Build history of the part. All positions in model axes, mm. Face numbers are marked on the shaded views. A direction names the side the tool comes from. Give positions to 0.01 mm unless a question says otherwise; leave off trailing zeros. Order: outer loops, then holes, each group sorted by start corner. A loop starts at its lowest first (then second) coordinate and runs counter-clockwise, first axis right, second up. Notation, with made-up numbers: (44, 34.5) -> (65, 34.5) arc R14 cw to (65, 43.5) -> close; hole circle Ø7 at (6.5, 60). An arc over 180 degrees is marked (long way). One line per question, with ' | ' between items. Start each with the question number.
(1) Pull direction X, two halves, no side cores. Call the marked faces 1, 2 and 3: +X half, -X half, draft (parallel to the pull), parting line (faces both ways), or undercut.
(2) Cut at C-C (y = -140). Give the cut face in (x, z), then the cut area to 3 significant figures.
(3) Drill centre lines: L1, parallel to Z at x = 10, y = -161; L2, parallel to Z at x = -1, y = -193.5. Where is each one in solid material? Low to high. Write a range as from..to.
(4) Pin check, flat tip, straight feed: pin 1 Ø2 at (x, z) = (-4, 16) entering from +Y. Stop position of the tip, or through.
(5) Which spindle directions (+Z, -Z, +X, -X, +Y, -Y) get a long thin tool onto all of the face, cutting with end or side? Do the marked faces 4 and 5. Say none if no direction does.
(6) Cut at A-A (z = 2). Give the cut face in (x, y).
(7) Cut at B-B (x = -8). Give the cut face in (y, z), then the cut area to 3 significant figures.
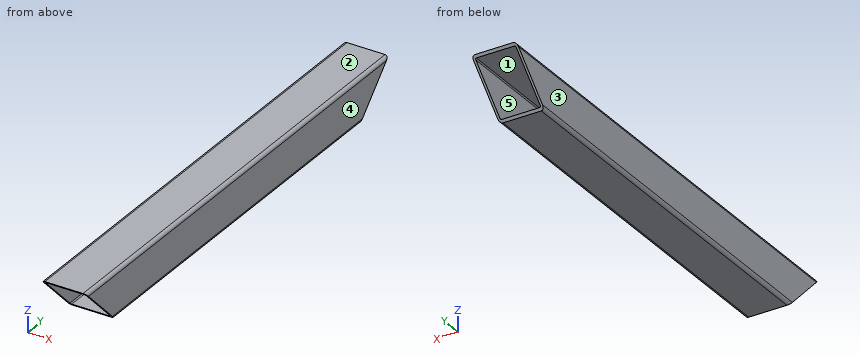
from build123d import *

# Parameters (mm, degrees)
F2_W     = 40
F2_H     = 40
F3_DEPTH = 214
F4_R     = 3
F5_T     = -2
F7_DEPTH = 40.001
F9_DEPTH = 40.001


with BuildPart() as f3:
    # F2 (on Front) → F3 (new body, symmetric)
    with BuildSketch(Plane.XZ):
        Rectangle(F2_W, F2_H)
    extrude(amount=F3_DEPTH, both=True)

    # F4
    f4_edges = [f3.edges().sort_by_distance(p)[0] for p in [
        (20, 0, 20),
        (-20, 0, 20),
        (20, 0, -20),
        (-20, 0, -20),
    ]]
    fillet(f4_edges, radius=F4_R)

    # F5
    f5_openings = [f3.faces().sort_by_distance(p)[0] for p in [
        (0, -214, 0),
        (0, 214, 0),
    ]]
    offset(amount=F5_T, openings=f5_openings)

    # F6 (on face) → F7 (cut, through all)
    with BuildSketch(Plane(origin=(-20, 0, 0), x_dir=(0, -1, 0), z_dir=(-1, 0, 0))):
        Polygon((-214, 20), (-214, -20), (-174, -20), align=None)
    extrude(amount=-F7_DEPTH, mode=Mode.SUBTRACT)

    # F8 (on face) → F9 (cut, through all)
    with BuildSketch(Plane.YZ.offset(20)):
        Polygon((-214, -20), (-174, -20), (-214, 20), align=None)
    extrude(amount=-F9_DEPTH, mode=Mode.SUBTRACT)


solid = f3.part
Result set:
1) face 1: undercut | face 2: draft | face 3: -X half
2) outline: (-20, -17) arc R3 ccw to (-17, -20) -> (17, -20) arc R3 ccw to (20, -17) -> (20, 17) arc R3 ccw to (17, 20) -> (-17, 20) arc R3 ccw to (-20, 17) -> close; hole (-18, -17) arc R1 ccw to (-17, -18) -> (17, -18) arc R1 ccw to (18, -17) -> (18, 17) arc R1 ccw to (17, 18) -> (-17, 18) arc R1 ccw to (-18, 17) -> close | area: 297 mm2
3) L1: z = -20..-18, 18..20 | L2: z = 18..20
4) pin 1: passes through
5) face 4: +Z, -Z, +X, +Y, -Y | face 5: +Y, -Y
6) outline: (-20, -196) -> (-18, -196) -> (-18, 196) -> (-20, 196) -> close; (18, -196) -> (20, -196) -> (20, 196) -> (18, 196) -> close
7) outline: (-214, 20) -> (-212, 18) -> (212, 18) -> (214, 20) -> close; (-176, -18) -> (-174, -20) -> (174, -20) -> (176, -18) -> close | area: 1,550 mm2
